```python
from build123d import *

# Parameters (mm, degrees)
SZKIC2_W                    = 34
SZKIC2_H                    = 38
SZKIC2_W_2                  = 30
SZKIC2_H_2                  = 31
DODANIE_WYCI_GNI_CIE1_DEPTH = 17
SZKIC6_W                    = 30
SZKIC6_H                    = 5
WYTNIJ_WYCI_GNI_CIE1_DEPTH  = 17
SZKIC7_W                    = 34
SZKIC7_H                    = 17
DODANIE_WYCI_GNI_CIE2_DEPTH = 10
SZKIC8_R                    = 11
SZKIC8_R_2                  = 5.35
SZKIC8_W                    = 7
SZKIC8_H                    = 4.5
SZKIC8_W_2                  = 34
SZKIC8_H_2                  = 17
DODANIE_WYCI_GNI_CIE3_DEPTH = 10
DODANIE_WYCI_GNI_CIE4_START = 17.5
SZKIC10_R                   = 11
SZKIC10_R_2                 = 5.35
DODANIE_WYCI_GNI_CIE4_DEPTH = 17.5
DODANIE_WYCI_GNI_CIE5_START = -16
SZKIC11_R                   = 5.35
SZKIC11_R_2                 = 4.2
DODANIE_WYCI_GNI_CIE5_DEPTH = 16
SZKIC13_R                   = 1.6
WYTNIJ_WYCI_GNI_CIE2_DEPTH  = 10
DODANIE_WYCI_GNI_CIE6_REACH = 79.494
SFAZOWANIE1_SIZE            = 2
SFAZOWANIE2_SIZE            = 2
SFAZOWANIE3_SIZE            = 2
ZAOKR_GLENIE1_R             = 5


with BuildPart() as part:
    # Szkic2 → Dodanie-wyciągnięcie1 (new body)
    with BuildSketch(Plane(origin=(0, 0, 0), x_dir=(1, 0, 0), z_dir=(0, 1, 0))):
        Rectangle(SZKIC2_W, SZKIC2_H)
        with Locations((0, 1.5)):
            Rectangle(SZKIC2_W_2, SZKIC2_H_2, mode=Mode.SUBTRACT)
    extrude(amount=DODANIE_WYCI_GNI_CIE1_DEPTH)

    # Szkic6 → Wytnij-wyciągnięcie1 (cut)
    with BuildSketch(Plane(origin=(0, 0, 14), x_dir=(-1, 0, 0), z_dir=(0, 0, -1))):
        with Locations((0, 14.5)):
            Rectangle(SZKIC6_W, SZKIC6_H)
        with Locations((0, 2.5)):
            Rectangle(SZKIC6_W, SZKIC6_H)
    extrude(amount=-WYTNIJ_WYCI_GNI_CIE1_DEPTH, mode=Mode.SUBTRACT)

    # Szkic7 → Dodanie-wyciągnięcie2 (add)
    with BuildSketch(Plane(origin=(0, 0, -19), x_dir=(-1, 0, 0), z_dir=(0, 0, -1))):
        with Locations((0, 8.5)):
            Rectangle(SZKIC7_W, SZKIC7_H)
    extrude(amount=DODANIE_WYCI_GNI_CIE2_DEPTH)

    # Szkic8 → Dodanie-wyciągnięcie3 (add)
    # profile 1 of 4: a face of its own
    with BuildSketch(Plane(origin=(0, 0, -29), x_dir=(-1, 0, 0), z_dir=(0, 0, -1))):
        with Locations((-37.5, 6)):
            Circle(SZKIC8_R)
        with Locations((-37.5, 6)):
            Circle(SZKIC8_R_2, mode=Mode.SUBTRACT)
    # profile 2 of 4: a face of its own
    with BuildSketch(Plane(origin=(0, 0, -29), x_dir=(-1, 0, 0), z_dir=(0, 0, -1))):
        with BuildLine():
            Line((-24, 12.5), (-24, 17))
            Line((-24, 17), (-37.5, 17))
            ThreePointArc((-37.5, 17), (-29.721825407, 13.778174593), (-26.5, 6))
            ThreePointArc((-26.5, 6), (-26.621602105, 4.368908572), (-26.983719863, 2.773879716))
            Line((-26.983719863, 2.773879716), (-24, 12.5))
        make_face()
    # profile 3 of 4: a face of its own
    with BuildSketch(Plane(origin=(0, 0, -29), x_dir=(-1, 0, 0), z_dir=(0, 0, -1))):
        with Locations((-20.5, 14.75)):
            Rectangle(SZKIC8_W, SZKIC8_H)
    # profile 4 of 4: a face of its own
    with BuildSketch(Plane(origin=(0, 0, -29), x_dir=(-1, 0, 0), z_dir=(0, 0, -1))):
        with Locations((0, 8.5)):
            Rectangle(SZKIC8_W_2, SZKIC8_H_2)
    extrude(amount=DODANIE_WYCI_GNI_CIE3_DEPTH)

    # Szkic10 → Dodanie-wyciągnięcie4 (add)
    with BuildSketch(Plane.XY.offset(-29).offset(DODANIE_WYCI_GNI_CIE4_START)):
        with Locations((37.5, 6)):
            Circle(SZKIC10_R)
        with Locations((37.5, 6)):
            Circle(SZKIC10_R_2, mode=Mode.SUBTRACT)
    extrude(amount=-DODANIE_WYCI_GNI_CIE4_DEPTH)

    # Szkic11 → Dodanie-wyciągnięcie5 (add)
    with BuildSketch(Plane(origin=(0, 0, -39), x_dir=(-1, 0, 0), z_dir=(0, 0, -1)).offset(DODANIE_WYCI_GNI_CIE5_START)):
        with Locations(Location((-37.5, 6, 0), (0, 0, 180))):
            Circle(SZKIC11_R)
        with Locations((-37.5, 6)):
            Circle(SZKIC11_R_2, mode=Mode.SUBTRACT)
    extrude(amount=DODANIE_WYCI_GNI_CIE5_DEPTH)

    # Szkic13 → Wytnij-wyciągnięcie2 (cut)
    with BuildSketch(Plane.XY.offset(-11.5)):
        with Locations((37.5, 14)):
            Circle(SZKIC13_R)
        with Locations((45.5, 6)):
            Circle(SZKIC13_R)
        with Locations((37.5, -2)):
            Circle(SZKIC13_R)
        with Locations((29.5, 6)):
            Circle(SZKIC13_R)
    extrude(amount=-WYTNIJ_WYCI_GNI_CIE2_DEPTH, mode=Mode.SUBTRACT)

    # Dodanie-wyciągnięcie6: up to this face of the body (flat: up to its plane)
    dodanie_wyci_gni_cie6_end = Plane(part.part.faces().sort_by_distance((26.811126984, 6, -11.5))[0])
    # Szkic16 → Dodanie-wyciągnięcie6 (add, up to the picked face)
    with BuildSketch(Plane(origin=(0, 0, -39), x_dir=(-1, 0, 0), z_dir=(0, 0, -1)), mode=Mode.PRIVATE) as dodanie_wyci_gni_cie6_sk1:
        with BuildLine():
            ThreePointArc((-48.5, 6), (-45.278174593, 13.778174593), (-37.5, 17))
            Line((-37.5, 17), (-48.5, 17))
            Line((-48.5, 17), (-48.5, 6))
        make_face()
    dodanie_wyci_gni_cie6_tool1 = split(extrude(dodanie_wyci_gni_cie6_sk1.sketch, amount=-DODANIE_WYCI_GNI_CIE6_REACH, mode=Mode.PRIVATE), bisect_by=dodanie_wyci_gni_cie6_end, keep=Keep.BOTH, mode=Mode.PRIVATE)
    # Szkic16 → Dodanie-wyciągnięcie6 (add, up to the picked face)
    with BuildSketch(Plane(origin=(0, 0, -39), x_dir=(-1, 0, 0), z_dir=(0, 0, -1)), mode=Mode.PRIVATE) as dodanie_wyci_gni_cie6_sk2:
        with BuildLine():
            Line((-26.5, 6), (-26.5, 17))
            Line((-26.5, 17), (-37.5, 17))
            ThreePointArc((-37.5, 17), (-29.721825407, 13.778174593), (-26.5, 6))
        make_face()
    dodanie_wyci_gni_cie6_tool2 = split(extrude(dodanie_wyci_gni_cie6_sk2.sketch, amount=-DODANIE_WYCI_GNI_CIE6_REACH, mode=Mode.PRIVATE), bisect_by=dodanie_wyci_gni_cie6_end, keep=Keep.BOTH, mode=Mode.PRIVATE)
    # Szkic16 → Dodanie-wyciągnięcie6 (add, up to the picked face)
    with BuildSketch(Plane(origin=(0, 0, -39), x_dir=(-1, 0, 0), z_dir=(0, 0, -1)), mode=Mode.PRIVATE) as dodanie_wyci_gni_cie6_sk3:
        with BuildLine():
            Line((-26.5, -5), (-26.5, 4.350675726))
            Line((-26.5, 4.350675726), (-26.983719863, 2.773879716))
            ThreePointArc((-26.983719863, 2.773879716), (-30.96116689, -2.84554473), (-37.5, -5))
            Line((-37.5, -5), (-26.5, -5))
        make_face()
    dodanie_wyci_gni_cie6_tool3 = split(extrude(dodanie_wyci_gni_cie6_sk3.sketch, amount=-DODANIE_WYCI_GNI_CIE6_REACH, mode=Mode.PRIVATE), bisect_by=dodanie_wyci_gni_cie6_end, keep=Keep.BOTH, mode=Mode.PRIVATE)
    # Szkic16 → Dodanie-wyciągnięcie6 (add, up to the picked face)
    with BuildSketch(Plane(origin=(0, 0, -39), x_dir=(-1, 0, 0), z_dir=(0, 0, -1)), mode=Mode.PRIVATE) as dodanie_wyci_gni_cie6_sk4:
        with BuildLine():
            ThreePointArc((-37.5, -5), (-45.278174593, -1.778174593), (-48.5, 6))
            Line((-48.5, 6), (-48.5, -5))
            Line((-48.5, -5), (-37.5, -5))
        make_face()
    dodanie_wyci_gni_cie6_tool4 = split(extrude(dodanie_wyci_gni_cie6_sk4.sketch, amount=-DODANIE_WYCI_GNI_CIE6_REACH, mode=Mode.PRIVATE), bisect_by=dodanie_wyci_gni_cie6_end, keep=Keep.BOTH, mode=Mode.PRIVATE)
    # Szkic16 → Dodanie-wyciągnięcie6 (add, up to the picked face)
    with BuildSketch(Plane(origin=(0, 0, -39), x_dir=(-1, 0, 0), z_dir=(0, 0, -1)), mode=Mode.PRIVATE) as dodanie_wyci_gni_cie6_sk5:
        with BuildLine():
            Line((-26.5, 4.350675726), (-26.5, 6))
            ThreePointArc((-26.5, 6), (-26.621602105, 4.368908572), (-26.983719863, 2.773879716))
            Line((-26.983719863, 2.773879716), (-26.5, 4.350675726))
        make_face()
    dodanie_wyci_gni_cie6_tool5 = split(extrude(dodanie_wyci_gni_cie6_sk5.sketch, amount=-DODANIE_WYCI_GNI_CIE6_REACH, mode=Mode.PRIVATE), bisect_by=dodanie_wyci_gni_cie6_end, keep=Keep.BOTH, mode=Mode.PRIVATE)
    add(dodanie_wyci_gni_cie6_tool1.solids().sort_by(Axis((46.042953, 14.542953, -39), (0, 0, 1)))[0])
    add(dodanie_wyci_gni_cie6_tool2.solids().sort_by(Axis((28.957047, 14.542953, -39), (0, 0, 1)))[0])
    add(dodanie_wyci_gni_cie6_tool3.solids().sort_by(Axis((28.969303, -2.578828, -39), (0, 0, 1)))[0])
    add(dodanie_wyci_gni_cie6_tool4.solids().sort_by(Axis((46.042953, -2.542953, -39), (0, 0, 1)))[0])
    add(dodanie_wyci_gni_cie6_tool5.solids().sort_by(Axis((26.597113, 4.365237, -39), (0, 0, 1)))[0])

    # Sfazowanie1
    sfazowanie1_edges = [part.edges().sort_by_distance(p)[0] for p in [
        (48.5, 17, -25.25),
        (26.5, 17, -20.25),
        (48.5, -5, -25.25),
        (26.5, -5, -25.25),
    ]]
    chamfer(sfazowanie1_edges, length=SFAZOWANIE1_SIZE)

    # Sfazowanie2
    sfazowanie2_edges = [part.edges().sort_by_distance(p)[0] for p in [
        (17, 6.25, -39),
        (0, 0, -39),
        (-17, 8.5, -39),
    ]]
    chamfer(sfazowanie2_edges, length=SFAZOWANIE2_SIZE)

    # Sfazowanie3
    sfazowanie3_edges = [part.edges().sort_by_distance(p)[0] for p in [
        (19.5, 12.5, -39),
        (15.75, 17, -39),
        (47.5, 16, -39),
        (48.5, 6, -39),
        (47.5, -4, -39),
        (37.5, -5, -39),
        (27.5, -4, -39),
        (26.5, 0.675337863, -39),
        (25.25, 8.425337863, -39),
    ]]
    chamfer(sfazowanie3_edges, length=SFAZOWANIE3_SIZE)

    # Zaokrąglenie1
    zaokr_glenie1_edges = [part.edges().sort_by_distance(p)[0] for p in [
        (17, 6.25, -37),
        (-17, 8.5, -37),
    ]]
    fillet(zaokr_glenie1_edges, radius=ZAOKR_GLENIE1_R)


solid = part.part
```
Work out the finished part from the listing and answer in its coordinate system (mm). A direction names the side the tool comes from. Give positions to 0.01 mm unless a question says otherwise; leave off trailing zeros. Order: outer loops, then holes, each group sorted by start corner. A loop starts at its lowest first (then second) coordinate and runs counter-clockwise, first axis right, second up. Notation, with made-up numbers: (42.25, -20) - (53.25, -20) arc R17 ccw to (53.25, 8) - close; hole circle Ø4 at (-24, 20.25). An arc over 180 degrees is marked (long way). One line per item, written item: value. Start each with the question number.
1. Section B-B, the plane x = -6 is taken. Write down the section's boundary in (y, z).
2. Section C-C, the plane z = -8 is taken. Write down the section's boundary in (x, y), then the cut area to 3 significant figures.
3. Section D-D, the plane x = 21.5 is taken. Write down the section's boundary in (y, z).
4. Each of these flat-tipped pins is pushed along its axis until it touches: pin 1 Ø1 at (y, z) = (-2.5, -12) entering from -X; pin 2 Ø6 at (x, y) = (21, 10) entering from +Z; pin 3 Ø5 at (y, z) = (6.5, 7.5) entering from +X. Where does it stop, or does it pass through?
5. Section A-A, the plane z = -27 is taken. Write down the section's boundary in (x, y).
6. Consider line 1 (X direction, y = 11.5, z = 12); line 2 (Y direction, x = 45.5, z = -15); line 3 (Z direction, x = 5, y = 7.5). Determine where each line is inside the solid, lowest interval first.
7. For a pull along Y with two mould halves and no side action, classify faces 1 (the face through (16.63, 7.08, -36.82)), 2 (the face through (37, 14, -21.5)), 3 (the face through (15, 16, -38)) as released by +Y, released by -Y, zero draft, split by the parting line, or undercut.
8. Which of the six approach directions +Z, -Z, +X, -X, +Y, -Y give full straight-line access (tool end or side, diameter ignored) to faces 4 (the face through (4, 0, -21)), 5 (the face through (26.5, 6, -22)), 6 (the face through (32, 9, -11.5)), 7 (the face through (0, 12, 16)), 8 (the face through (36.32, -0.92, -16.43))?
Filled sheet:
1. outline: (0, -37) - (2, -39) - (15, -39) - (17, -37) - (17, -17) - (0, -17) - close; (5, 14) - (12, 14) - (12, 19) - (5, 19) - close
2. outline: (-17, 0) - (-15, 0) - (-15, 17) - (-17, 17) - close; (15, 0) - (17, 0) - (17, 17) - (15, 17) - close
2. area: 68.0 mm²
3. outline: (12.5, -37) - (14.5, -39) - (15, -39) - (17, -37) - (17, -29) - (12.5, -29) - close
4. pin 1: x = 26.5
4. pin 2: z = -29
4. pin 3: x = 17
5. outline: (-17, 0) - (17, 0) - (17, 17) - (-17, 17) - close; (26.5, -3) - (28.5, -5) - (46.5, -5) - (48.5, -3) - (48.5, 15) - (46.5, 17) - (28.5, 17) - (26.5, 15) - close; hole circle Ø8.4 at (37.5, 6)
6. line 1: -17 to -15, 15 to 17
6. line 2: -5 to 4.4, 7.6 to 17
6. line 3: -39 to -17, 14 to 19
7. face 1: zero draft
7. face 2: undercut
7. face 3: released by +Y
8. face 4: +Z, -Z, -X, -Y
8. face 5: +Z, -Y
8. face 6: +Z, +X, +Y, -Y
8. face 7: +Z, +Y
8. face 8: +Z
